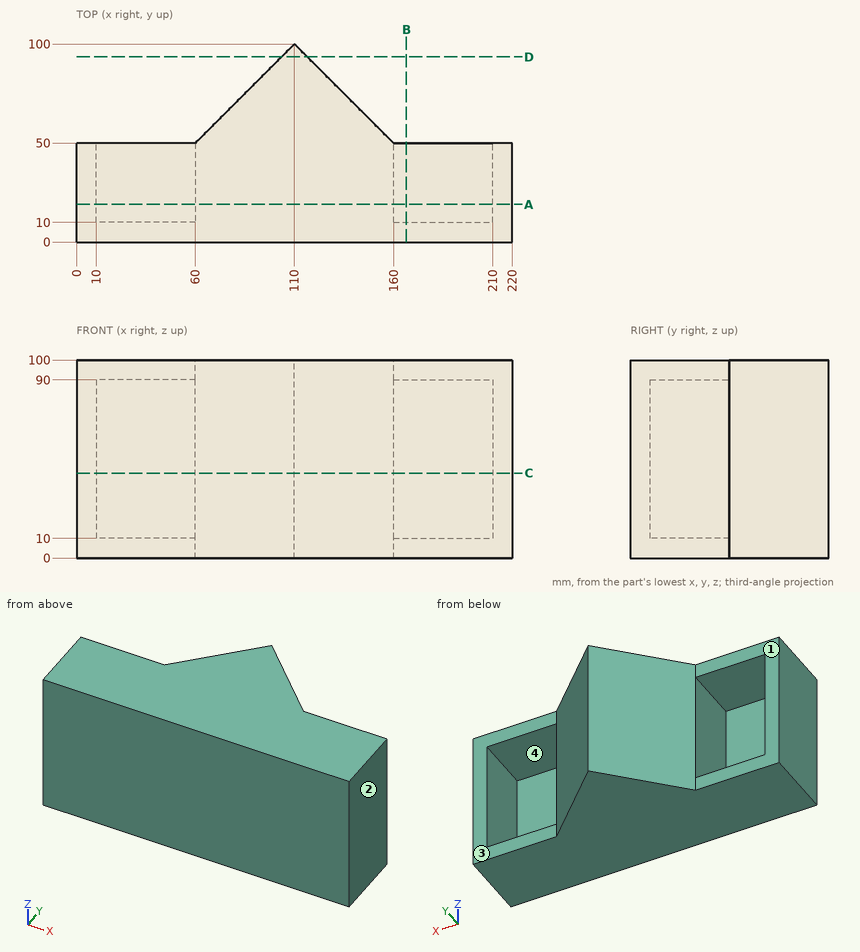
Geometry check sheet. Reference: drawing and pictorial views, mm from the part's lowest x, y, z. A direction names the side the tool comes from. Round coordinates to 2 decimals unless told otherwise and drop trailing zeros. Loops run counter-clockwise (first coordinate to the right, second up) from the corner with the lowest first, then second, coordinate; pieces in that order, holes last. Notation, with made-up numbers: (8, 36) - (19, 36) arc R20 ccw to (19, 66) - close; hole circle Ø1 at (23.25, 1). An arc over 180 degrees is marked (long way). Write item = value, one per line. Start each with the question number.
Q1. Section check C-C (z = 43). Record the boundary of the cut face in (x, y), plus the area to 3 significant figures.
Q2. Section check A-A (y = 19). Record the boundary of the cut face in (x, z), plus the area to 3 significant figures.
Q3. Section check B-B (x = 166.5). Record the boundary of the cut face in (y, z), plus the area to 3 significant figures.
Q4. Section check D-D (y = 93.5). Record the boundary of the cut face in (x, z), plus the area to 3 significant figures.
Q5. Thickness scan on L1, parallel to X at y = 15, z = 87.5; L2, parallel to Z at x = 195, y = 43; L3, parallel to Y at x = 196.5, z = 72. Record the ranges inside material, lowest first.
Q6. Access from +Z, -Z, +X, -X, +Y, -Y to the whole of each face (thin tool, end or side, straight path). Record for the marked faces 1, 2, 3 and 4.
Q7. Depth check by flat-ended pin: P1, Ø6, axis at y = 75, z = 15, coming from the +X side; P2, Ø1.5, axis at y = 89, z = 50.5, coming from the +X side; P3, Ø1.5, axis at y = 59.5, z = 24.5, coming from the +X side. Enter the tip coordinate at first touch or a pass-through.
Derived:
q1.outline = (0, 0) - (220, 0) - (220, 50) - (210, 50) - (210, 10) - (160, 10) - (160, 50) - (110, 100) - (60, 50) - (60, 10) - (10, 10) - (10, 50) - (0, 50) - close
q1.area = 9,500 mm^2
q2.outline = (0, 0) - (220, 0) - (220, 100) - (0, 100) - close; hole (10, 10) - (60, 10) - (60, 90) - (10, 90) - close; hole (160, 10) - (210, 10) - (210, 90) - (160, 90) - close
q2.area = 14,000 mm^2
q3.outline = (0, 0) - (50, 0) - (50, 10) - (10, 10) - (10, 90) - (50, 90) - (50, 100) - (0, 100) - close
q3.area = 1,800 mm^2
q4.outline = (103.5, 0) - (116.5, 0) - (116.5, 100) - (103.5, 100) - close
q4.area = 1,300 mm^2
q5.L1 = 0 to 10, 60 to 160, 210 to 220
q5.L2 = 0 to 10, 90 to 100
q5.L3 = 0 to 10
q6.face_1 = +Z, -Z, -X, +Y
q6.face_2 = +Z, -Z, +X, +Y, -Y
q6.face_3 = +Z, -Z, +X, +Y
q6.face_4 = +Y
q7.P1 = 138
q7.P2 = 121.75
q7.P3 = 151.25
